```python
from build123d import *

# Parameters (mm, degrees)
SKETCH1_R           = 1.6
BOSS_EXTRUDE1_DEPTH = 3
SKETCH2_W           = 4.751236483
SKETCH2_H           = 10.264254991
BOSS_EXTRUDE2_DEPTH = 2.6
SKETCH3_R           = 1.118711993
CUT_EXTRUDE1_DEPTH  = 4.751236483
SKETCH4_R           = 1.769310005
CUT_EXTRUDE2_DEPTH  = 5
SKETCH6_R           = 4
BOSS_EXTRUDE3_DEPTH = 20.2
SKETCH7_R           = 2.25
CUT_EXTRUDE3_DEPTH  = 8
FILLET1_R           = 2


with BuildPart() as part:
    # Sketch1 → Boss-Extrude1 (new body)
    with BuildSketch(Plane.XY):
        with BuildLine():
            Line((0, 2.5), (36.470564138, 2.5))
            Line((36.470564138, 2.5), (36.470564138, -3.124783652))
            Line((36.470564138, -3.124783652), (29.945161274, -3.124783652))
            Line((29.945161274, -3.124783652), (29.945161274, 0.647373355))
            Line((29.945161274, 0.647373355), (26.216359637, 0.647373355))
            Line((26.216359637, 0.647373355), (26.216359637, -9.893369232))
            Line((26.216359637, -9.893369232), (-2.5, -9.447534254))
            Line((-2.5, -9.447534254), (-2.5, 0))
            ThreePointArc((-2.5, 0), (-1.767766953, 1.767766953), (0, 2.5))
        make_face()
        Circle(SKETCH1_R, mode=Mode.SUBTRACT)
    extrude(amount=BOSS_EXTRUDE1_DEPTH)

    # Sketch2 → Boss-Extrude2 (add)
    with BuildSketch(Plane.XY.offset(3)):
        with Locations((23.840741396, -4.761241737)):
            Rectangle(SKETCH2_W, SKETCH2_H)
    extrude(amount=BOSS_EXTRUDE2_DEPTH)

    # Sketch3 → Cut-Extrude1 (cut)
    with BuildSketch(Plane(origin=(26.216359637, 0, 0), x_dir=(0, 0, -1), z_dir=(1, 0, 0))):
        with Locations((-3.241173045, -5.729114241)):
            Circle(SKETCH3_R)
    extrude(amount=-CUT_EXTRUDE1_DEPTH, mode=Mode.SUBTRACT)

    # Sketch4 → Cut-Extrude2 (cut)
    with BuildSketch(Plane(origin=(0, 0, 0), x_dir=(-1, 0, 0), z_dir=(0, 0, -1))):
        with Locations((-33, 0)):
            Circle(SKETCH4_R)
    extrude(amount=-CUT_EXTRUDE2_DEPTH, mode=Mode.SUBTRACT)

    # Sketch6 → Boss-Extrude3 (add)
    with BuildSketch(Plane.XY.offset(3)):
        with Locations((7.967965429, -4.6419924)):
            Circle(SKETCH6_R)
    extrude(amount=BOSS_EXTRUDE3_DEPTH)

    # Sketch7 → Cut-Extrude3 (cut)
    with BuildSketch(Plane.XY.offset(23.2)):
        with Locations((7.967965429, -4.6419924)):
            Circle(SKETCH7_R)
    extrude(amount=-CUT_EXTRUDE3_DEPTH, mode=Mode.SUBTRACT)

    # Fillet1
    fillet1_edges = [part.edges().sort_by_distance(p)[0] for p in [
        (36.470564138, 2.5, 1.5),
        (36.470564138, -3.124783652, 1.5),
        (29.945161274, -3.124783652, 1.5),
        (-2.5, -9.447534254, 1.5),
    ]]
    fillet(fillet1_edges, radius=FILLET1_R)


solid = part.part
```
Input: part model. Units: mm. Frame: model coordinates. A direction names the side the tool comes from. Round coordinates to 2 decimals unless told otherwise and drop trailing zeros. Loops run counter-clockwise (first coordinate to the right, second up) from the corner with the lowest first, then second, coordinate; pieces in that order, holes last. Notation, with made-up numbers: (-21, 71) -> (-5, 71) arc R19 ccw to (-5, 99) -> close; hole circle Ø9 at (59, 34.25). An arc over 180 degrees is marked (long way). Use one line per item in the form item = value. Start each with the question number.
Item 1: Contact query for flat-ended pins moving along their axis: pin 1 Ø2 at (x, y) = (26.5, -4) entering from -Z; pin 2 Ø3 at (y, z) = (1, 5) entering from -X; pin 3 Ø0.8 at (x, z) = (33, 1.5) entering from -Y; pin 4 Ø3.5 at (x, y) = (16.5, -4.5) entering from +Z. Output: stop coordinate, or through.
Item 2: Set-up query: faces 4 (the face through (26.216, -5, 2)), 5 (the face through (24, -5, 5.6)), 6 (the face through (8, -5, 15.2)), 7 (the face through (23.87, -6.41, 4.13)). Return all of +Z, -Z, +X, -X, +Y, -Y with unobstructed straight access to the full face (end or side cutting, diameter ignored); none if empty.
Item 3: Section query A-A on x = 33. Return the cut outline in (y, z), then the cut area to 3 significant figures.
Item 4: Mould query, pull axis X, two halves, no side actions, for faces 1 (the face through (30.547, -2.554, 1.521)), 2 (the face through (13, -4, 0)), 3 (the face through (35.9, 1.9, 1.5)). Classes: pulls with the +X half, pulls with the -X half, needs draft (parallel to the pull), parting line crosses it, or undercut.
Item 5: Section query D-D on x = 15. Return the cut outline in (y, z).
Item 6: Material intervals for L1, parallel to Y at x = 33, z = 1.45; L2, parallel to Y at x = 0, z = 2.3; L3, parallel to Z at x = 12, y = -1, sorted ascending. Write a range as from..to.
Item 7: Section query B-B on x = 22. Return the cut outline in (y, z).
Item 8: Section query C-C on z = 6.25. Return the cut outline in (x, y).
Ans:
q1.pin_1 = 0
q1.pin_2 = 21.47
q1.pin_3 = -3.12
q1.pin_4 = 3
q2.face_4 = +Z, -Z, -Y
q2.face_5 = +Z, +X, +Y, -Y
q2.face_6 = +Z
q2.face_7 = +X
q3.outline = (-3.12, 0) -> (-1.77, 0) -> (-1.77, 3) -> (-3.12, 3) -> close; (1.77, 0) -> (2.5, 0) -> (2.5, 3) -> (1.77, 3) -> close
q3.area = 6.26 mm^2
q4.face_1 = undercut
q4.face_2 = needs draft
q4.face_3 = pulls with the +X half
q5.outline = (-9.72, 0) -> (2.5, 0) -> (2.5, 3) -> (-9.72, 3) -> close
q6.L1 = -3.12..-1.77, 1.77..2.5
q6.L2 = -9.49..-1.6, 1.6..2.5
q6.L3 = 0..3
q7.outline = (-9.89, 3) -> (-9.83, 3) -> (-9.83, 0) -> (2.5, 0) -> (2.5, 3) -> (0.37, 3) -> (0.37, 5.6) -> (-9.89, 5.6) -> close; hole circle Ø2.24 at (-5.73, 3.24)
q8.outline = circle Ø8 at (7.97, -4.64)
